Build history of the part. All positions in model axes, mm. A direction names the side the tool comes from. Give positions to 0.01 mm unless a question says otherwise; leave off trailing zeros. Write each loop counter-clockwise with the first axis right and the second up, starting at its lowest first coordinate (ties: lowest second). Pieces come first, ordered by that corner, then holes. Notation, with made-up numbers: (77.5, -16) -> (86.5, -16) arc R8 cw to (86.5, -4) -> close; hole circle Ø3 at (-29.5, 67). An arc over 180 degrees is marked (long way). Put each result on its own line as item: value. Start each with the question number.
Item 1: Slice it at B-B, the plane x = -3.5. List the corners of the cut face in (y, z), plus the area to 3 significant figures.
Item 2: Flat gauge pins, fed straight in: pin 1 Ø1.8 at (x, z) = (57.29, -35.04) entering from +Y; pin 2 Ø2 at (x, y) = (-52.5, 1.5) entering from +Z; pin 3 Ø2 at (y, z) = (0.5, -1) entering from -X; pin 4 Ø0.6 at (x, y) = (-12, 1) entering from -Z. Where does each tip first touch, or does it go through?
Item 3: Slice it at D-D, the plane z = 31. List the corners of the cut face in (x, y).
Item 4: Slice it at C-C, the plane z = 8. List the corners of the cut face in (x, y).
Item 5: Slice it at A-A, the plane y = 0.6. List the corners of the cut face in (x, z), plus the area to 3 significant figures.
Item 6: Two-plate mould, pull along X, no slides. Class faces 1 (the cylindrical face through (54.664, 0.986, 31.269)), 2 (the cylindrical face through (55.96, -0.99, 34.65)), 3 (the flat face through (-53, 2, -1)), 4 (the cylindrical face through (55.96, -0.99, -34.35)): pulls with the +X half, pulls with the -X half, needs draft (parallel to the pull), parting line crosses it, or undercut.
Item 7: Tool access for faces 5 (the cylindrical face through (54.6, 0.99, -32.42)), 6 (the cylindrical face through (-57.085, 0.986, 31.269)), 7 (the cylindrical face through (-57.02, 0.99, -32.42)), 8 (the cylindrical face through (-61.04, -0.99, -34.35)), 9 (the flat face through (-2, -2, -1)): list every direction of +Z, -Z, +X, -X, +Y, -Y with a clear straight run to the whole face (end or side of a thin tool).
Item 8: Drill centre lines: line 1 along X through (y, z) = (1.4, -28); line 2 along X through (y, z) = (1.7, 32); line 3 along Z through (x, y) = (5, 0.8). Where is each one in solid material? Low to high.
```python
from build123d import *

# Parameters (mm, degrees)
EXTRUDE_1_DEPTH     = 2
EXTRUDE_2_DEPTH     = 2
SKETCH_1_5_W        = 123
SKETCH_1_5_H        = 75
EXTRUDE_3_DEPTH     = 2
SKETCH_1_6_R        = 1.5
CUT_EXTRUDE_1_DEPTH = 12


with BuildPart() as part:
    # Sketch 1 → Extrude 1 (new body)
    with BuildSketch(Plane(origin=(0, 0, 0), x_dir=(1, 0, 0), z_dir=(0, 1, 0))):
        with BuildLine():
            Line((-46.710495983, 35.042327972), (-55.294297496, 35.042327972))
            ThreePointArc((-55.294297496, 35.042327972), (-57.053641733, 32.385473722), (-59.710495983, 30.626129484))
            Line((-59.710495983, 30.626129484), (-59.710495983, -29.541473541))
            ThreePointArc((-59.710495983, -29.541473541), (-57.053641733, -31.300817779), (-55.294297496, -33.957672028))
            Line((-55.294297496, -33.957672028), (-46.710495983, -33.957672028))
            Line((-46.710495983, -33.957672028), (-46.710495983, 35.042327972))
        make_face()
    extrude(amount=EXTRUDE_1_DEPTH)



with BuildPart() as body_2:
    # Sketch 1_4 → Extrude 2 (new body)
    with BuildSketch(Plane(origin=(0, 0, 0), x_dir=(1, 0, 0), z_dir=(0, 1, 0))):
        with BuildLine():
            Line((-43.710495983, 35.042327972), (52.87330553, 35.042327972))
            ThreePointArc((52.87330553, 35.042327972), (54.632649768, 32.385473722), (57.289504017, 30.626129484))
            Line((57.289504017, 30.626129484), (57.289504017, -29.541473541))
            ThreePointArc((57.289504017, -29.541473541), (54.632649768, -31.300817779), (52.87330553, -33.957672028))
            Line((52.87330553, -33.957672028), (-43.710495983, -33.957672028))
            Line((-43.710495983, -33.957672028), (-43.710495983, 35.042327972))
        make_face()
    extrude(amount=EXTRUDE_2_DEPTH)


with BuildPart() as part_1:
    add(part.part)

    add(body_2.part)  # Extrude 3 merges body 2
    # Sketch 1_5 → Extrude 3 (add)
    with BuildSketch(Plane(origin=(0, 0, 0), x_dir=(1, 0, 0), z_dir=(0, 1, 0))):
        with Locations((-1.210495983, 0.542327972)):
            Rectangle(SKETCH_1_5_W, SKETCH_1_5_H)
    extrude(amount=-EXTRUDE_3_DEPTH)

    # Sketch 1_6 → Cut-Extrude 1 (cut)
    with BuildSketch(Plane(origin=(0, 0, 0), x_dir=(1, 0, 0), z_dir=(0, 1, 0))):
        with Locations(Location((-59.710495983, 35.042327972, 0), (0, 0, 270))):
            Circle(SKETCH_1_6_R)
        with Locations(Location((-59.710495983, -33.957672028, 0), (0, 0, 270))):
            Circle(SKETCH_1_6_R)
        with Locations(Location((57.289504017, -33.957672028, 0), (0, 0, 270))):
            Circle(SKETCH_1_6_R)
        with Locations(Location((57.289504017, 35.042327972, 0), (0, 0, 270))):
            Circle(SKETCH_1_6_R)
    extrude(amount=-CUT_EXTRUDE_1_DEPTH, mode=Mode.SUBTRACT)


solid = part_1.part
```
Values follow:
1. outline: (-2, -38.04) -> (0, -38.04) -> (0, -35.04) -> (2, -35.04) -> (2, 33.96) -> (0, 33.96) -> (0, 36.96) -> (-2, 36.96) -> close
1. area: 288 mm2
2. pin 1: through
2. pin 2: z = 33.96
2. pin 3: x = -62.71
2. pin 4: z = -35.04
3. outline: (-62.71, -2) -> (60.29, -2) -> (60.29, 0) -> (54.95, 0) -> (54.95, 2) -> (-43.71, 2) -> (-43.71, 0) -> (-46.71, 0) -> (-46.71, 2) -> (-57.37, 2) -> (-57.37, 0) -> (-62.71, 0) -> close
4. outline: (-62.71, -2) -> (60.29, -2) -> (60.29, 0) -> (57.29, 0) -> (57.29, 2) -> (-43.71, 2) -> (-43.71, 0) -> (-46.71, 0) -> (-46.71, 2) -> (-59.71, 2) -> (-59.71, 0) -> (-62.71, 0) -> close
5. outline: (-59.71, -30.63) arc R8 cw to (-55.29, -35.04) -> (-46.71, -35.04) -> (-46.71, 33.96) -> (-55.29, 33.96) arc R8 cw to (-59.71, 29.54) -> close; (-43.71, -35.04) -> (52.87, -35.04) arc R8 cw to (57.29, -30.63) -> (57.29, 29.54) arc R8 cw to (52.87, 33.96) -> (-43.71, 33.96) -> close
5. area: 7,820 mm2
6. face 1: pulls with the +X half
6. face 2: undercut
6. face 3: needs draft
6. face 4: undercut
7. face 5: -Z, +X, +Y
7. face 6: +Z, -X, +Y
7. face 7: -Z, -X, +Y
7. face 8: +Y, -Y
7. face 9: +Z, -Z, +X, -X, -Y
8. line 1: -59.71 to -46.71, -43.71 to 57.29
8. line 2: -56.43 to -46.71, -43.71 to 54.01
8. line 3: -35.04 to 33.96
